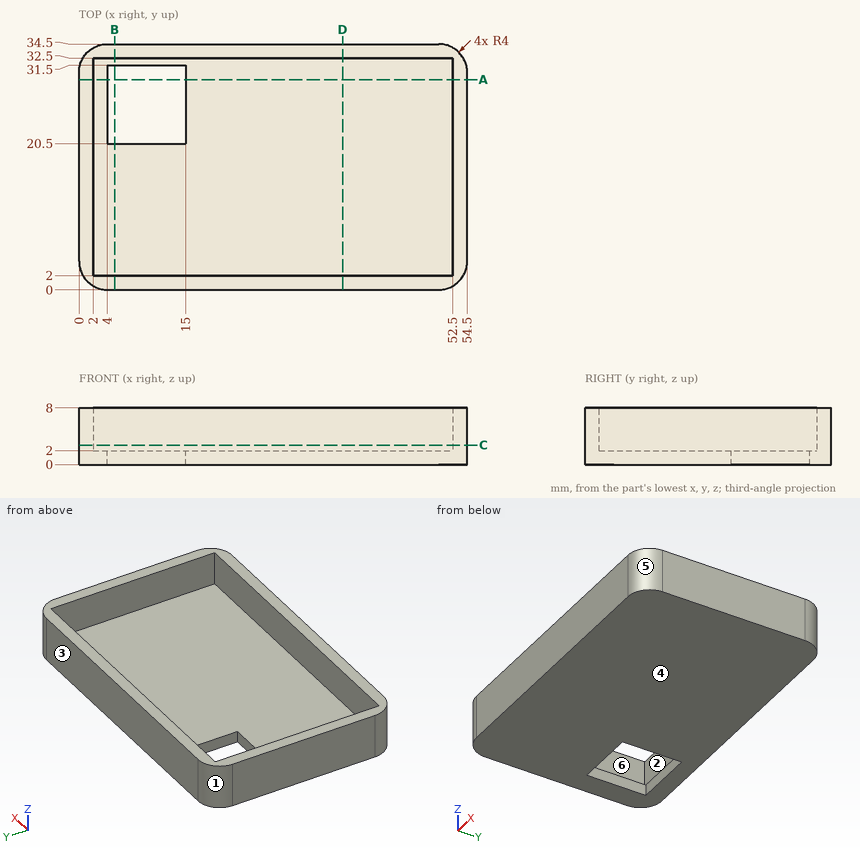
Print and shaded views of the part. All mm, measured from the part's lowest x, y and z. A direction names the side the tool comes from. Give positions to 0.01 mm unless a question says otherwise; leave off trailing zeros. Loops run counter-clockwise (first coordinate to the right, second up) from the corner with the lowest first, then second, coordinate; pieces in that order, holes last. Notation, with made-up numbers: (76, -12.75) -> (84, -12.75) arc R23 cw to (84, 8.25) -> close; hole circle Ø6 at (84.5, 83.5). An arc over 180 degrees is marked (long way). Use a Markdown table: item, result.
1. Slice it at C-C (z = 2.75). List the corners of the cut face in (x, y).
Check result:
| item | result |
|---|---|
| outline | (0, 4) arc R4 ccw to (4, 0) -> (50.5, 0) arc R4 ccw to (54.5, 4) -> (54.5, 30.5) arc R4 ccw to (50.5, 34.5) -> (4, 34.5) arc R4 ccw to (0, 30.5) -> close; hole (2, 2) -> (52.5, 2) -> (52.5, 32.5) -> (2, 32.5) -> close |
2. Slice it at D-D (x = 37). List the corners of the cut face in (y, z).
Check result:
| item | result |
|---|---|
| outline | (0, 0) -> (34.5, 0) -> (34.5, 8) -> (32.5, 8) -> (32.5, 2) -> (2, 2) -> (2, 8) -> (0, 8) -> close |
3. Flat gauge pin, fed straight in: pin 1 (4 mm diameter, centred on x = 6, y = 17, fed in from +Z). Where does the tip first touch, or does it go through?
Check result:
| item | result |
|---|---|
| pin 1 | stops at z = 2 |
4. Wall check: L1, parallel to X at y = 29, z = 0.5; L2, parallel to X at y = 30, z = 3.5; L3, parallel to Y at x = 10, z = 3.75. Give the ranges that are in metal, low to high. Write a range as [from, to].
Check result:
| item | result |
|---|---|
| L1 | x = [0, 4], [15, 54.5] |
| L2 | x = [0, 2], [52.5, 54.5] |
| L3 | y = [0, 2], [32.5, 34.5] |
5. Which spindle directions (+Z, -Z, +X, -X, +Y, -Y) get a long thin tool onto all of the face, cutting with end or side? Do the marked faces 1 and 2. Say none if no direction does.
Check result:
| item | result |
|---|---|
| face 1 | +Z, -Z, -X, +Y |
| face 2 | +Z |
6. Slice it at A-A (y = 29.5). List the corners of the cut face in (x, z), plus the area to 3 significant figures.
Check result:
| item | result |
|---|---|
| outline | (0, 0) -> (4, 0) -> (4, 2) -> (2, 2) -> (2, 8) -> (0, 8) -> close; (15, 0) -> (54.5, 0) -> (54.5, 8) -> (52.5, 8) -> (52.5, 2) -> (15, 2) -> close |
| area | 111 mm^2 |
7. Mould opens along Y. For the marked faces 3, 4, 5 and 6 say: pulls with the +Y half, pulls with the -Y half, needs draft (parallel to the pull), parting line crosses it, or undercut.
Check result:
| item | result |
|---|---|
| face 3 | pulls with the +Y half |
| face 4 | needs draft |
| face 5 | pulls with the -Y half |
| face 6 | undercut |
8. Slice it at B-B (x = 5). List the corners of the cut face in (y, z).
Check result:
| item | result |
|---|---|
| outline | (0, 0) -> (20.5, 0) -> (20.5, 2) -> (2, 2) -> (2, 8) -> (0, 8) -> close; (31.5, 0) -> (34.5, 0) -> (34.5, 8) -> (32.5, 8) -> (32.5, 2) -> (31.5, 2) -> close |
